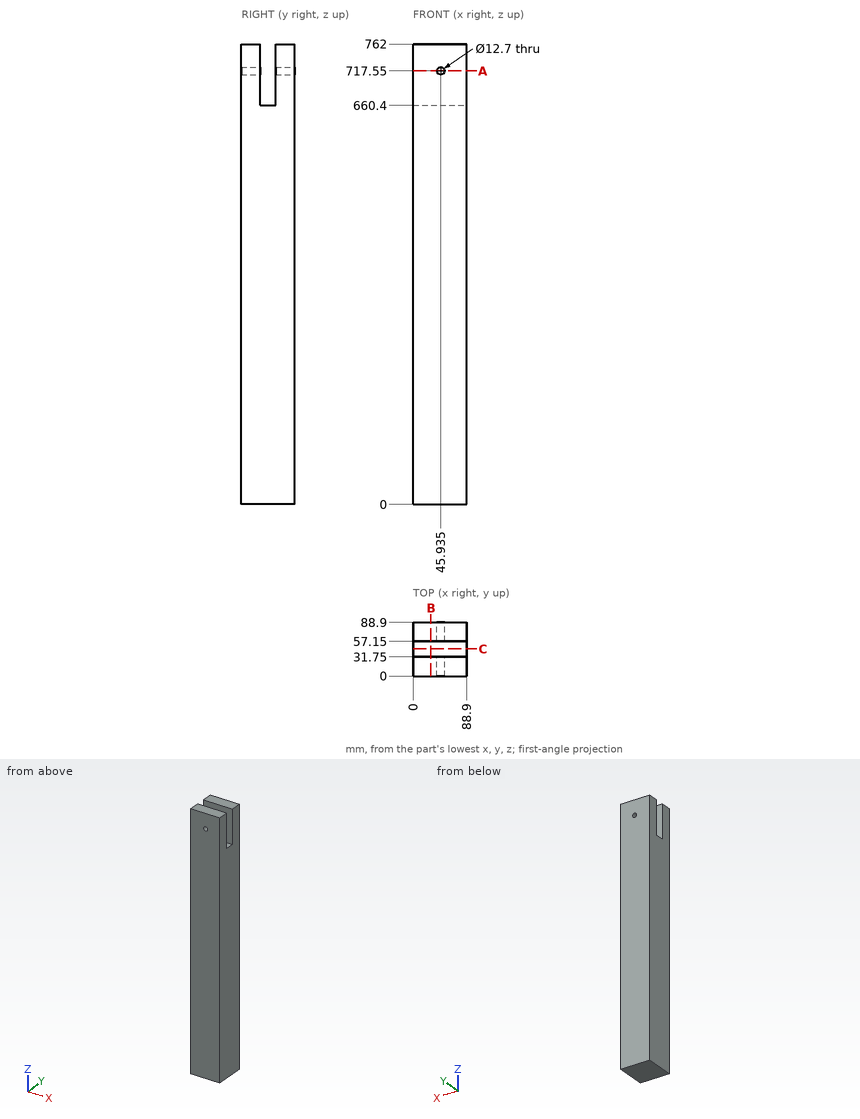
Verification items for this drawing (mm, ordinates from the low corner). Coordinates: 2 decimals unless noted, no trailing zeros. Loops run counter-clockwise (first coordinate to the right, second up) from the corner with the lowest first, then second, coordinate; pieces in that order, holes last. Notation, with made-up numbers: (-5, 45.25) -> (43, 45.25) arc R8 ccw to (43, 53.25) -> close; hole circle Ø11 at (10, 81.5). An arc over 180 degrees is marked (long way). Answer in a Markdown table with one row per item. Add a question column.
1. Depth check by flat-ended pin: P1, Ø7.5, axis at x = 39.5, y = 46.5, coming from the +Z side; P2, Ø7.5, axis at x = 45.93, z = 717.55, coming from the +Y side. Enter the tip coordinate at first touch or a pass-through.
2. Section check B-B, the plane x = 29.5. Enter the section's corners in (y, z).
3. Section check A-A, the plane z = 717.55. Give the number of separate pieces and of enclosed holes in the cut face, then the cut area to 3 significant figures.
4. Section check C-C, the plane y = 45. Enter the section's corners in (x, z), then the cut area to 3 significant figures.
5. Material ranges on probe 1 along X at (y, z) = (21, 717.55) (1 decimal); probe 2 along Y at (x, z) = (71, 704); probe 3 along Z at (x, y) = (45, 11), recorded low to high. Write a range as [from, to].
Derived:
| question | item | result |
|---|---|---|
| 1 | P1 | stops at z = 660.4 |
| 1 | P2 | passes through |
| 2 | outline | (0, 0) -> (88.9, 0) -> (88.9, 762) -> (57.15, 762) -> (57.15, 660.4) -> (31.75, 660.4) -> (31.75, 762) -> (0, 762) -> close |
| 3 | separate pieces | 4 |
| 3 | enclosed holes | 0 |
| 3 | area | 4,840 mm² |
| 4 | outline | (0, 0) -> (88.9, 0) -> (88.9, 660.4) -> (0, 660.4) -> close |
| 4 | area | 58,700 mm² |
| 5 | probe 1 | x = [0, 39.6], [52.3, 88.9] |
| 5 | probe 2 | y = [0, 31.75], [57.15, 88.9] |
| 5 | probe 3 | z = [0, 711.27], [723.83, 762] |
